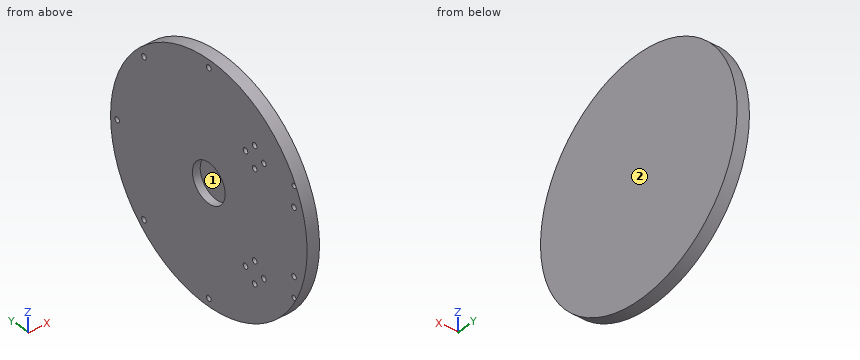
from build123d import *

# Parameters (mm, degrees)
SKETCH_1_R          = 12.5
SKETCH_1_R_2        = 1.75
EXTRUDE_1_DEPTH     = 5
FILLET_1_R          = 5
SKETCH_3_R          = 1.1
CUT_EXTRUDE_2_DEPTH = 10
SKETCH_4_R          = 1.5
CUT_EXTRUDE_3_DEPTH = 10
EXTRUDE1_DEPTH      = 311.885831134
SKETCH2_R           = 75
EXTRUDE2_DEPTH      = 3


with BuildPart() as part:
    # 草图1 → 凸台-拉伸1 (new body)
    with BuildSketch(Plane(origin=(0, 0, 0), x_dir=(0, 0, -1), z_dir=(1, 0, 0))):
        with BuildLine():
            Line((0, 0), (0, 160))
            ThreePointArc((0, 160), (60, 280), (120, 160))
            Line((120, 160), (120, 0))
            Line((120, 0), (0, 0))
        make_face()
        with Locations((60, 205)):
            Circle(SKETCH_1_R, mode=Mode.SUBTRACT)
        with Locations((25, 177)):
            Circle(SKETCH_1_R_2, mode=Mode.SUBTRACT)
        with Locations((32, 170)):
            Circle(SKETCH_1_R_2, mode=Mode.SUBTRACT)
        with Locations((25, 163)):
            Circle(SKETCH_1_R_2, mode=Mode.SUBTRACT)
        with Locations((18, 170)):
            Circle(SKETCH_1_R_2, mode=Mode.SUBTRACT)
        with Locations((95, 177)):
            Circle(SKETCH_1_R_2, mode=Mode.SUBTRACT)
        with Locations((102, 170)):
            Circle(SKETCH_1_R_2, mode=Mode.SUBTRACT)
        with Locations((95, 163)):
            Circle(SKETCH_1_R_2, mode=Mode.SUBTRACT)
        with Locations((88, 170)):
            Circle(SKETCH_1_R_2, mode=Mode.SUBTRACT)
        with Locations((39, 140)):
            Circle(SKETCH_1_R_2, mode=Mode.SUBTRACT)
        with Locations((81, 140)):
            Circle(SKETCH_1_R_2, mode=Mode.SUBTRACT)
        with Locations((60, 275)):
            Circle(SKETCH_1_R_2, mode=Mode.SUBTRACT)
        with Locations((-10, 205)):
            Circle(SKETCH_1_R_2, mode=Mode.SUBTRACT)
        with Locations((130, 205)):
            Circle(SKETCH_1_R_2, mode=Mode.SUBTRACT)
        with Locations((10.502525317, 254.497474683)):
            Circle(SKETCH_1_R_2, mode=Mode.SUBTRACT)
        with Locations((109.497474683, 254.497474683)):
            Circle(SKETCH_1_R_2, mode=Mode.SUBTRACT)
        with Locations((5, 5)):
            Circle(SKETCH_1_R_2, mode=Mode.SUBTRACT)
        with Locations((115, 5)):
            Circle(SKETCH_1_R_2, mode=Mode.SUBTRACT)
        with Locations((5, 120)):
            Circle(SKETCH_1_R_2, mode=Mode.SUBTRACT)
        with Locations((115, 120)):
            Circle(SKETCH_1_R_2, mode=Mode.SUBTRACT)
        with BuildLine():
            Line((40.5, 81), (40.5, 59))
            ThreePointArc((40.5, 59), (39, 57.5), (37.5, 59))
            Line((37.5, 59), (37.5, 81))
            ThreePointArc((37.5, 81), (39, 82.5), (40.5, 81))
        make_face(mode=Mode.SUBTRACT)
        with BuildLine():
            Line((79.5, 81), (79.5, 59))
            ThreePointArc((79.5, 59), (81, 57.5), (82.5, 59))
            Line((82.5, 59), (82.5, 81))
            ThreePointArc((82.5, 81), (81, 82.5), (79.5, 81))
        make_face(mode=Mode.SUBTRACT)
    extrude(amount=EXTRUDE_1_DEPTH)

    # 圆角1
    fillet_1_edges = [part.edges().sort_by_distance(p)[0] for p in [
        (2.5, 0, 0),
        (2.5, 160, 0),
        (2.5, 160, -120),
        (2.5, 0, -120),
    ]]
    fillet(fillet_1_edges, radius=FILLET_1_R)

    # 草图3 → 切除-拉伸2 (cut)
    with BuildSketch(Plane.ZY):
        with Locations((-45.818141739, 127.45827935)):
            Circle(SKETCH_3_R)
        with Locations((-61.818141739, 127.45827935)):
            Circle(SKETCH_3_R)
        with Locations((-45.818141739, 91.45827935)):
            Circle(SKETCH_3_R)
        with Locations((-61.818141739, 91.45827935)):
            Circle(SKETCH_3_R)
        with BuildLine():
            Line((-20, 46.75), (-30, 46.75))
            ThreePointArc((-30, 46.75), (-31.75, 48.5), (-30, 50.25))
            Line((-30, 50.25), (-20, 50.25))
            ThreePointArc((-20, 50.25), (-18.25, 48.5), (-20, 46.75))
        make_face()
        with BuildLine():
            Line((-90, 46.75), (-100, 46.75))
            ThreePointArc((-100, 46.75), (-101.75, 48.5), (-100, 50.25))
            Line((-100, 50.25), (-90, 50.25))
            ThreePointArc((-90, 50.25), (-88.25, 48.5), (-90, 46.75))
        make_face()
        with BuildLine():
            Line((-20, 8.25), (-30, 8.25))
            ThreePointArc((-30, 8.25), (-31.75, 10), (-30, 11.75))
            Line((-30, 11.75), (-20, 11.75))
            ThreePointArc((-20, 11.75), (-18.25, 10), (-20, 8.25))
        make_face()
        with BuildLine():
            Line((-90, 8.25), (-100, 8.25))
            ThreePointArc((-100, 8.25), (-101.75, 10), (-100, 11.75))
            Line((-100, 11.75), (-90, 11.75))
            ThreePointArc((-90, 11.75), (-88.25, 10), (-90, 8.25))
        make_face()
    extrude(amount=-CUT_EXTRUDE_2_DEPTH, mode=Mode.SUBTRACT)

    # 草图4 → 切除-拉伸3 (cut)
    with BuildSketch(Plane.ZY):
        with Locations((-16.118918229, 88.740617872)):
            Circle(SKETCH_4_R)
        with Locations((-16.118918229, 64.240617872)):
            Circle(SKETCH_4_R)
        with Locations((-94, 140)):
            Circle(SKETCH_4_R)
        with Locations((-26, 140)):
            Circle(SKETCH_4_R)
        with Locations((-94, 82)):
            Circle(SKETCH_4_R)
        with Locations((-26, 82)):
            Circle(SKETCH_4_R)
    extrude(amount=-CUT_EXTRUDE_3_DEPTH, mode=Mode.SUBTRACT)

    # Sketch1 → Extrude1 (cut, through all)
    with BuildSketch(Plane.ZY):
        with BuildLine():
            Line((0.9375, 161.277910689), (0.9375, -17.17747431))
            Line((0.9375, -17.17747431), (-120, -17.17747431))
            Line((-120, -17.17747431), (-120.9375, 161.277910689))
            ThreePointArc((-120.9375, 161.277910689), (-60, 130), (0.9375, 161.277910689))
        make_face()
    extrude(amount=-EXTRUDE1_DEPTH, mode=Mode.SUBTRACT)

    # Sketch2 → Extrude2 (add)
    with BuildSketch(Plane(origin=(5, 0, 0), x_dir=(0, 0, -1), z_dir=(1, 0, 0))):
        with Locations(Location((60, 205, 0), (0, 0, 180))):
            Circle(SKETCH2_R)
    extrude(amount=EXTRUDE2_DEPTH)


solid = part.part
The model under review builds one solid part; all positions refer to its coordinate system, in mm. Face numbers are marked on the shaded views. Give positions to 0.01 mm unless a question says otherwise; leave off trailing zeros. Order: outer loops, then holes, each group sorted by start corner. A loop starts at its lowest first (then second) coordinate and runs counter-clockwise, first axis right, second up. Notation, with made-up numbers: M 68,35 L 73,35 A31 cw 73,61 Z; hole C 38,47 d2. An arc over 180 degrees is marked long. Answer in a Markdown table with one row per item. Add a question column.
1. Mouldability with a two-part tool opening along Z and no side actions: class the marked faces 1 and 2 as released by +Z, released by -Z, zero draft, split by the parting line, or undercut.
2. To check wall thickness, follow line 1 along Z through (x, y) = (1.3, 170); line 2 along Y through (x, z) = (2.25, -25); line 3 along Z through (x, y) = (1.5, 140). State the ranges of each line that lie inside material, in increasing order.
3. For pin 1 Ø4 at (x, z) = (5, -17.5) entering from +Y; pin 2 Ø1 at (y, z) = (254.5, -109) entering from -X; pin 3 Ø4 at (x, z) = (7, -41.5) entering from +Y, all flat-tipped, find the tip position at first contact; note any pin that passes through.
4. Add section C-C on y = 170. State the section outline as (x, z) points.
5. Add section D-D on z = -102. State the section outline as (x, y) points.
6. Add section A-A on x = 3.75. Count the separate pieces of the cut face and the enclosed holes in it, plus the area to 3 significant figures.
7. Add section B-B on z = -60. State the section outline as (x, y) points.
The answers:
| question | item | result |
|---|---|---|
| 1 | face 1 | undercut |
| 1 | face 2 | zero draft |
| 2 | line 1 | -126.33 to -103.75, -100.25 to -89.75, -86.25 to -33.75, -30.25 to -19.75, -16.25 to 6.33 |
| 2 | line 2 | 138.67 to 138.88, 141.12 to 161.25, 164.75 to 175.25, 178.75 to 271.33 |
| 2 | line 3 | -97.42 to -95.5, -92.5 to -82.75, -79.25 to -40.75, -37.25 to -27.5, -24.5 to -22.58 |
| 3 | pin 1 | y = 268.12 |
| 3 | pin 2 | x = 5 |
| 3 | pin 3 | y = 278.16 |
| 4 | outline | M 0,-126.33 L 8,-126.33 L 8,6.33 L 0,6.33 L 0,-16.25 L 5,-16.25 L 5,-19.75 L 0,-19.75 L 0,-30.25 L 5,-30.25 L 5,-33.75 L 0,-33.75 L 0,-86.25 L 5,-86.25 L 5,-89.75 L 0,-89.75 L 0,-100.25 L 5,-100.25 L 5,-103.75 L 0,-103.75 Z |
| 5 | outline | M 0,142.86 L 8,142.86 L 8,267.14 L 0,267.14 L 0,171.75 L 5,171.75 L 5,168.25 L 0,168.25 Z |
| 6 | separate pieces | 1 |
| 6 | enclosed holes | 18 |
| 6 | area | 17,000 mm2 |
| 7 | outline | M 0,130 L 8,130 L 8,280 L 0,280 L 0,276.75 L 5,276.75 L 5,273.25 L 0,273.25 L 0,217.5 L 5,217.5 L 5,192.5 L 0,192.5 Z |
